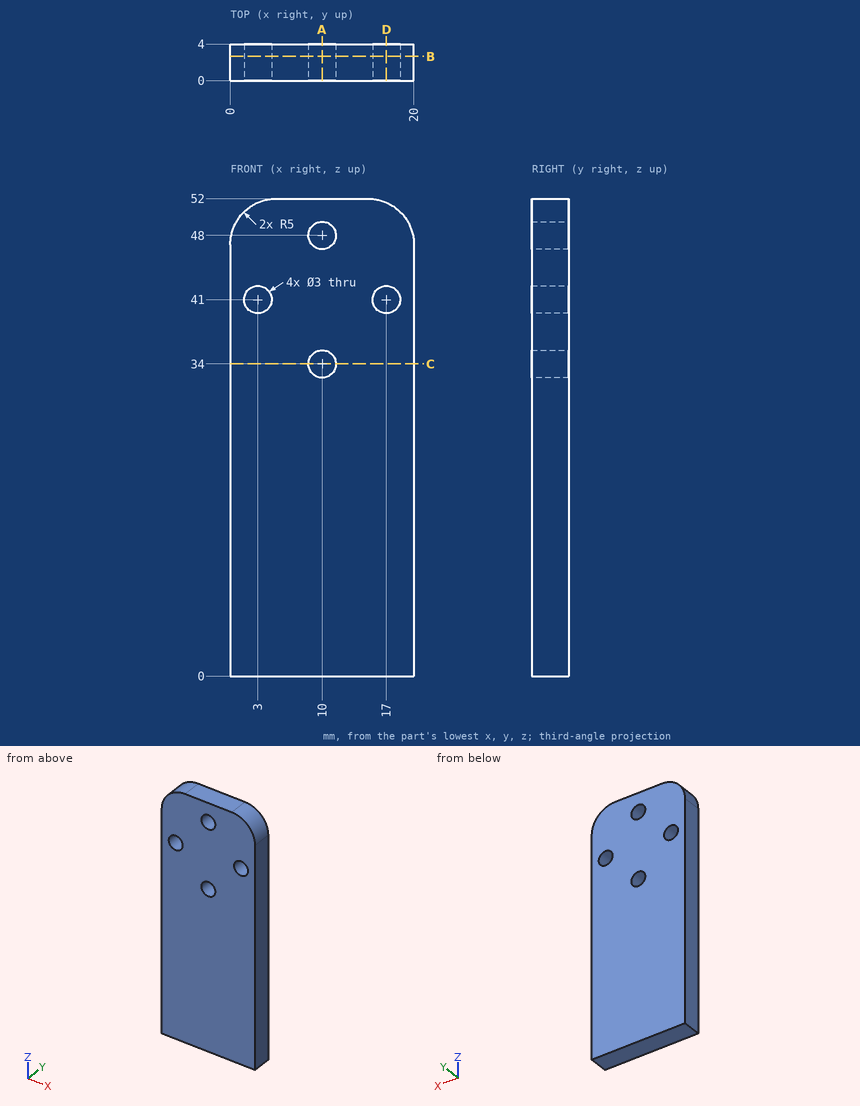
Check sheet for the drawn part. Datum: minimum x, y, z corner. Units: mm. Round coordinates to 2 decimals unless told otherwise and drop trailing zeros. Loops run counter-clockwise (first coordinate to the right, second up) from the corner with the lowest first, then second, coordinate; pieces in that order, holes last. Notation, with made-up numbers: M -15,31 L 28,31 A7 cw 28,36 Z; hole C 54,0.5 d6. An arc over 180 degrees is marked long. One line per question, with ' | ' between items. Start each with the question number.
Item 1: Gauge pin test, flat end, axial feed: pin 1 Ø4 at (x, z) = (10, 34) entering from -Y. Record the tip position at first contact, or that the pin passes through.
Item 2: Section check A-A (x = 10). Record the boundary of the cut face in (y, z), and give its area (3 significant figures).
Item 3: Scan lines: probe 1 along X at (y, z) = (1.35, 41); probe 2 along X at (y, z) = (1.55, 34); probe 3 along X at (y, z) = (1.55, 48). Record each from-to range of solid material in increasing order.
Item 4: Section check D-D (x = 17). Record the boundary of the cut face in (y, z), and give its area (3 significant figures).
Item 5: Section check B-B (y = 2.65). Record the boundary of the cut face in (x, z), and give its area (3 significant figures).
Item 6: Section check C-C (z = 34). Record the boundary of the cut face in (x, y).
Worked out:
1) pin 1: y = 0
2) outline: M 0,0 L 4,0 L 4,32.5 L 0,32.5 Z; M 0,35.5 L 4,35.5 L 4,46.5 L 0,46.5 Z; M 0,49.5 L 4,49.5 L 4,52 L 0,52 Z | area: 184 mm^2
3) probe 1: 0 to 1.5, 4.5 to 15.5, 18.5 to 20 | probe 2: 0 to 8.5, 11.5 to 20 | probe 3: 0.1 to 8.5, 11.5 to 19.9
4) outline: M 0,0 L 4,0 L 4,39.5 L 0,39.5 Z; M 0,42.5 L 4,42.5 L 4,51.58 L 0,51.58 Z | area: 194 mm^2
5) outline: M 0,0 L 20,0 L 20,47 A5 ccw 15,52 L 5,52 A5 ccw 0,47 Z; hole C 3,41 d3; hole C 10,34 d3; hole C 10,48 d3; hole C 17,41 d3 | area: 1,000 mm^2
6) outline: M 0,0 L 8.5,0 L 8.5,4 L 0,4 Z; M 11.5,0 L 20,0 L 20,4 L 11.5,4 Z
